```python
from build123d import *

# Parameters (mm, degrees)
F0_R     = 6.1870864942
F0_R_2   = 3.8241120886
F2_DEPTH = 10
F3_R     = 4.5894677587
F4_DEPTH = 3.7


with BuildPart() as f2:
    # F0 (on Top) → F2 (new body)
    with BuildSketch(Plane.XY):
        with BuildLine():
            Line((33.4636883251, 43.2611741126), (13.4636883251, 43.2611741126))
            Line((13.4636883251, 43.2611741126), (13.4636883251, 27.7164801955))
            Line((13.4636883251, 27.7164801955), (13.4636883251, 23.0237431824))
            ThreePointArc((13.4636883251, 23.0237431824), (23.4636883251, 13.0237431824), (33.4636883251, 23.0237431824))
            Line((33.4636883251, 23.0237431824), (33.4636883251, 43.2611741126))
        make_face()
        with Locations((23.4636883251, 23.0237431824)):
            Circle(F0_R, mode=Mode.SUBTRACT)
        with Locations((23.4636883251, 23.0237431824)):
            Circle(F0_R)
        with Locations((23.4636883251, 23.0237431824)):
            Circle(F0_R_2, mode=Mode.SUBTRACT)
    extrude(amount=F2_DEPTH)

    # F3 (on Top) → F4 (cut)
    with BuildSketch(Plane.XY):
        with Locations((23.3934633434, 22.9011047632)):
            Circle(F3_R)
    extrude(amount=F4_DEPTH, mode=Mode.SUBTRACT)


solid = f2.part
```
Geometry check sheet. Reference: the model listing, model coordinates, mm. A direction names the side the tool comes from. Coordinates: 2 decimals unless noted, no trailing zeros. Order: outer loops, then holes, each group sorted by start corner. A loop starts at its lowest first (then second) coordinate and runs counter-clockwise, first axis right, second up.
Q1. Sectioned sample at D-D on y = 16. Record the cut outline in (x, z).
Reply:
outline: (16.35, 0) - (30.58, 0) - (30.58, 10) - (16.35, 10) - close
Q2. Sectioned sample at C-C on z = 5.25. Record the cut outline in (x, y).
Reply:
outline: (13.46, 23.02) arc R10 ccw to (33.46, 23.02) - (33.46, 43.26) - (13.46, 43.26) - close; hole circle Ø7.65 at (23.46, 23.02)
Q3. Depth check by flat-ended pin: pin 1 Ø7 at (x, y) = (23.46, 23.02) entering from -Z. Enter the tip coordinate at first touch or a pass-through.
Reply:
pin 1: passes through
Q4. Draft check along Y on faces 1 (the face through (24, 43.261, 5)), 2 (the face through (23, 28, 0)), 3 (the face through (25.51, 18.83, 1.82)). Enter one of: released by +Y, released by -Y, zero draft, split by the parting line, or undercut.
Reply:
face 1: released by +Y
face 2: zero draft
face 3: undercut
Q5. Thickness scan on probe 1 along X at (y, z) = (25, 4.75); probe 2 along Y at (x, z) = (24.25, 1.5); probe 3 along X at (y, z) = (22, 7). Record the ranges inside material, lowest first.
Reply:
probe 1: x = 13.46 to 20.19, 26.74 to 33.46
probe 2: y = 13.05 to 18.39, 27.41 to 43.26
probe 3: x = 13.52 to 19.78, 27.15 to 33.41
Q6. Sectioned sample at B-B on y = 26.5. Record the cut outline in (x, z).
Reply:
outline: (13.46, 0) - (20.55, 0) - (20.55, 3.7) - (21.87, 3.7) - (21.87, 10) - (13.46, 10) - close; (25.06, 3.7) - (26.24, 3.7) - (26.24, 0) - (33.46, 0) - (33.46, 10) - (25.06, 10) - close
Q7. Sectioned sample at A-A on x = 24. Record the cut outline in (y, z), and give its area (3 significant figures).
Reply:
outline: (13.04, 0) - (18.35, 0) - (18.35, 3.7) - (19.24, 3.7) - (19.24, 10) - (13.04, 10) - close; (26.81, 3.7) - (27.45, 3.7) - (27.45, 0) - (43.26, 0) - (43.26, 10) - (26.81, 10) - close
area: 221 mm2
Q8. Tool access check on faces 4 (the face through (23.244, 13.026, 4.93)), 5 (the face through (23, 19, 3.7)). Record the directions out of +Z, -Z, +X, -X, +Y, -Y that give a thin tool (end or side, any length) a straight path to the whole face; none if there is none.
Reply:
face 4: +Z, -Z, -Y
face 5: -Z
